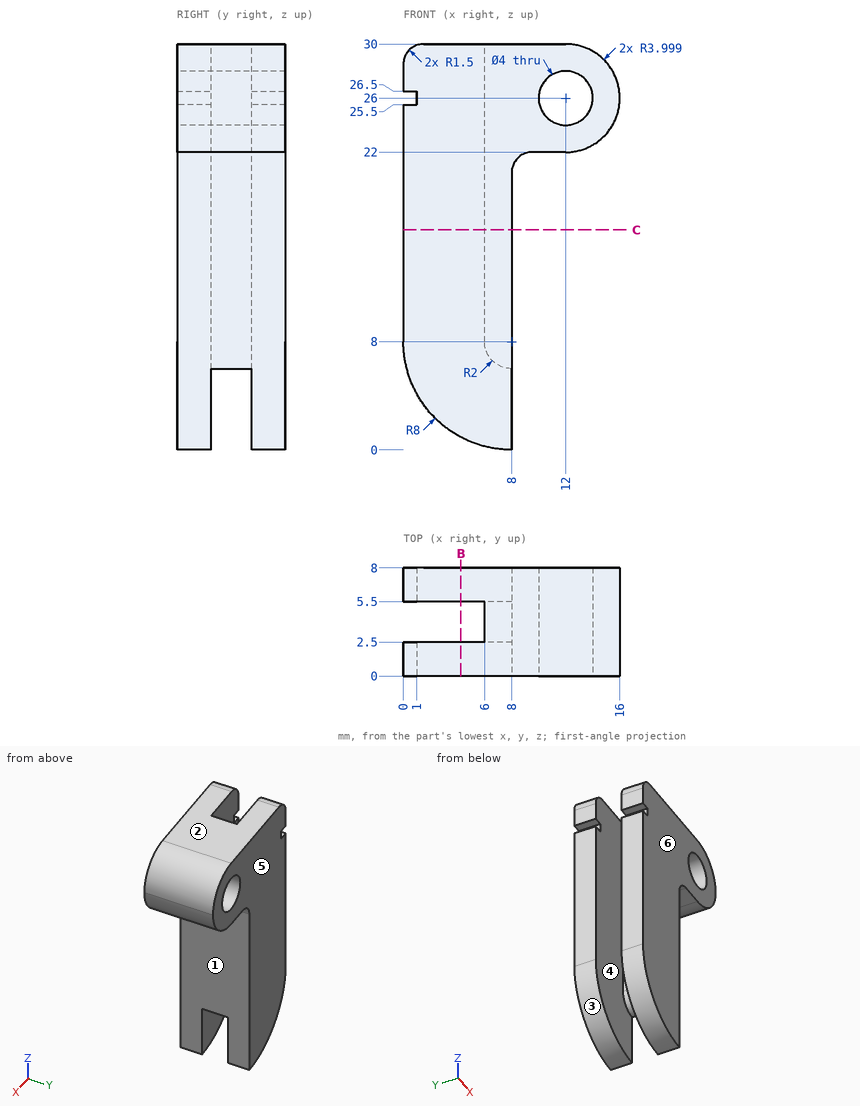
Input: dimensioned drawing with shaded views. Units: mm. Origin: part minimum x, y, z. A direction names the side the tool comes from. Coordinates: 2 decimals unless noted, no trailing zeros. Order: outer loops, then holes, each group sorted by start corner. A loop starts at its lowest first (then second) coordinate and runs counter-clockwise, first axis right, second up.
(1) Material intervals for probe 1 along Y at (x, z) = (5.75, 9.5); probe 2 along X at (y, z) = (2, 26); probe 3 along X at (y, z) = (5.25, 26), sorted ascending.
(2) Section query C-C (z = 16.25). Return the cut outline in (x, y).
(3) Access query for the marked faces 1 and 2. Directions: +Z, -Z, +X, -X, +Y, -Y. A direction counts if a zero-diameter tool reaches every point of the face in a straight line with its end or side. Return the directions, or none.
(4) First-contact query: pin 1 (0.8 mm diameter, centred on y = 7, z = 26, fed in from -X); pin 2 (1.5 mm diameter, centred on x = 6, y = 3.5, fed in from -Z); pin 3 (2 mm diameter, centred on x = 11.5, y = 6, fed in from -Z). Flat tips, straight axial feed; report the tip coordinate or a pass-through.
(5) Section query B-B (x = 4.25). Return the cut outline in (y, z).
(6) Draft query along Y for the marked faces 3, 4, 5 and 6. Return one class per face: pulls with the +Y half, pulls with the -Y half, needs draft (parallel to the pull), parting line crosses it, or undercut.
Solution:
1. probe 1: y = 0 to 2.5, 5.5 to 8
1. probe 2: x = 1 to 10, 14 to 16
1. probe 3: x = 6 to 10, 14 to 16
2. outline: (0, 0) - (8, 0) - (8, 8) - (0, 8) - (0, 5.5) - (6, 5.5) - (6, 2.5) - (0, 2.5) - close
3. face 1: -Z, +X, +Y, -Y
3. face 2: +Z, +X, -X, +Y, -Y
4. pin 1: stops at x = 1
4. pin 2: stops at z = 6.44
4. pin 3: stops at z = 22
5. outline: (0, 0.93) - (2.5, 0.93) - (2.5, 30) - (0, 30) - close; (5.5, 0.93) - (8, 0.93) - (8, 30) - (5.5, 30) - close
6. face 3: needs draft
6. face 4: undercut
6. face 5: pulls with the +Y half
6. face 6: pulls with the -Y half
